```python
from build123d import *

# Parameters (mm, degrees)
BOSS_EXTRUDE1_DEPTH = 29.5
CUT_EXTRUDE1_REACH  = 132
SKETCH2_W           = 5
SKETCH2_H           = 5
SKETCH3_W           = 1.8
SKETCH3_H           = 1.8
BOSS_EXTRUDE2_DEPTH = 130
FILLET1_R           = 3
FILLET2_R           = 1
FILLET3_R           = 0.25


with BuildPart() as part:
    # Sketch1 → Boss-Extrude1 (new body)
    with BuildSketch(Plane.XY):
        Polygon((0, 0), (0, 26), (130, 26), (130, 20), (6, 20), (6, 0), align=None)
    extrude(amount=BOSS_EXTRUDE1_DEPTH)

    # Sketch2 → Cut-Extrude1 (cut, up to next)
    with BuildSketch(Plane.ZY, mode=Mode.PRIVATE) as cut_extrude1_sk1:
        with Locations((14.75, 2.5)):
            Rectangle(SKETCH2_W, SKETCH2_H)
    cut_extrude1_tool1 = extrude(cut_extrude1_sk1.sketch, amount=-CUT_EXTRUDE1_REACH, mode=Mode.PRIVATE) & part.part
    add(cut_extrude1_tool1.solids().sort_by_distance((0, 2.5, 14.75))[0], mode=Mode.SUBTRACT)

    # Sketch3 → Boss-Extrude2 (add)
    with BuildSketch(Plane.ZY):
        with Locations((-0.9, 23)):
            Rectangle(SKETCH3_W, SKETCH3_H)
        with Locations((30.4, 23)):
            Rectangle(SKETCH3_W, SKETCH3_H)
    extrude(amount=-BOSS_EXTRUDE2_DEPTH)

    # Fillet1
    fillet1_edges = [part.edges().sort_by_distance(p)[0] for p in [
        (0, 26, 14.75),
    ]]
    fillet(fillet1_edges, radius=FILLET1_R)

    # Fillet2
    fillet2_edges = [part.edges().sort_by_distance(p)[0] for p in [
        (3, 5, 17.25),
        (3, 0, 17.25),
        (3, 0, 12.25),
        (3, 5, 12.25),
        (0, 2.5, 17.25),
        (0, 5, 14.75),
        (0, 2.5, 12.25),
    ]]
    fillet(fillet2_edges, radius=FILLET2_R)

    # Fillet3
    fillet3_edges = [part.edges().sort_by_distance(p)[0] for p in [
        (65, 22.1, -1.8),
        (65.069091198, 23.9, -1.8),
        (65.069091198, 23.9, 31.3),
        (65, 22.1, 31.3),
    ]]
    fillet(fillet3_edges, radius=FILLET3_R)


solid = part.part
```
For this review, take the finished solid that the model builds, in its own axes (mm). A direction names the side the tool comes from. Coordinates: 2 decimals unless noted, no trailing zeros. Loops run counter-clockwise (first coordinate to the right, second up) from the corner with the lowest first, then second, coordinate; pieces in that order, holes last.
1. Mouldability with a two-part tool opening along Z and no side actions: class faces 1 (the flat face through (6, 10, 15)), 2 (the flat face through (3, 2, 12.25)), 3 (the flat face through (51, 21, 0)) as +Z half, -Z half, draft (parallel to the pull), parting line (faces both ways), or undercut.
2. For faces 4 (the flat face through (66, 25, 29.5)), 5 (the flat face through (3, 2, 17.25)), 6 (the flat face through (66, 25, 0)), list the 3-axis set-ups (+Z, -Z, +X, -X, +Y, -Y) from which the entire face can be reached by the end or side of a thin tool; tool diameter is ignored.
3. Add section C-C, the plane y = 18.5. Give the boundary of the cut face in (x, z), then the cut area to 3 significant figures.
4. For line 1 (X direction, y = 23.75, z = 7); line 2 (Y direction, x = 51.5, z = 25.5); line 3 (Z direction, x = 48, y = 20.5), list the stretches that pass through material, from the lowest coordinate up.
5. Add section A-A, the plane z = 2.5. Give the boundary of the cut face in (x, y), then the cut area to 3 significant figures.
6. Add section B-B, the plane x = 56. Give the boundary of the cut face in (y, z), then the cut area to 3 significant figures.
7. Add section D-D, the plane z = 15. Give the boundary of the cut face in (x, y).
8. Insertion check: P1, Ø12, axis at x = 97, z = 2.5, coming from the -Y side; P2, Ø0.6, axis at x = 89.5, y = 25, coming from the +Z side; P3, Ø1.7, axis at x = 94, z = 30.5, coming from the +Y side; P4, Ø6.5, axis at x = 93.5, y = 15.5, coming from the -Z side. Each pin has a flat end and moves straight along its axis. Give the tip position at first contact, or say it passes through.
Result:
1. face 1: draft
1. face 2: undercut
1. face 3: -Z half
2. face 4: +Z, +X, -X, +Y
2. face 5: +X, -X, -Y
2. face 6: -Z, +X, -X, +Y
3. outline: (0, 0) - (6, 0) - (6, 29.5) - (0, 29.5) - close
3. area: 177 mm2
4. line 1: x = 0.1 to 130
4. line 2: y = 20 to 26
4. line 3: z = 0 to 29.5
5. outline: (0, 0) - (6, 0) - (6, 20) - (130, 20) - (130, 26) - (3, 26) arc R3 ccw to (0, 23) - close
5. area: 898 mm2
6. outline: (20, 0) - (22.1, 0) - (22.1, -1.55) arc R0.25 ccw to (22.35, -1.8) - (23.65, -1.8) arc R0.25 ccw to (23.9, -1.55) - (23.9, 0) - (26, 0) - (26, 29.5) - (23.9, 29.5) - (23.9, 31.05) arc R0.25 ccw to (23.65, 31.3) - (22.35, 31.3) arc R0.25 ccw to (22.1, 31.05) - (22.1, 29.5) - (20, 29.5) - close
6. area: 183 mm2
7. outline: (0, 6) arc R1 ccw to (1, 5) - (6, 5) - (6, 20) - (130, 20) - (130, 26) - (3, 26) arc R3 ccw to (0, 23) - close
8. P1: stops at y = 20
8. P2: stops at z = 29.5
8. P3: stops at y = 23.9
8. P4: passes through
